```python
from build123d import *

# Parameters (mm, degrees)
ESBO_O2_R                = 1
RESSALTO_EXTRUS_O1_DEPTH = 1
RESSALTO_EXTRUS_O2_START = 1
ESBO_O4_R                = 1
RESSALTO_EXTRUS_O2_DEPTH = 1
CHANFRO1_SIZE            = 0.3
CHANFRO2_SIZE            = 0.3


with BuildPart() as part:
    # Esboço1 → Revolução2 (revolve)
    with BuildSketch(Plane.XY, mode=Mode.PRIVATE) as revolu_o2_sk:
        Polygon((-1, 5), (-1.5, 5), (-1.5, 0), (1.5, 0), (1.5, 5), (1, 5), (1, 4), (0, 4), (-1, 4), align=None)
    revolve(revolu_o2_sk.sketch.rotate(Axis((0, 0, 0), (1, 0, 0)), 90), axis=Axis((0, 0, 0), (1, 0, 0)))

    # Esboço2 → Ressalto-extrusão1 (add)
    with BuildSketch(Plane.ZY.offset(1.5)):
        Circle(ESBO_O2_R)
    extrude(amount=RESSALTO_EXTRUS_O1_DEPTH)

    # Esboço4 → Ressalto-extrusão2 (add)
    with BuildSketch(Plane(origin=(1.5, 0, 0), x_dir=(0, 0, -1), z_dir=(1, 0, 0)).offset(RESSALTO_EXTRUS_O2_START)):
        with Locations(Location((0, 0, 0), (0, 0, 180))):
            Circle(ESBO_O4_R)
    extrude(amount=-RESSALTO_EXTRUS_O2_DEPTH)

    # Chanfro1
    chanfro1_edges = [part.edges().sort_by_distance(p)[0] for p in [
        (-2.5, 0, -1),
    ]]
    chamfer(chanfro1_edges, length=CHANFRO1_SIZE)

    # Chanfro2
    chanfro2_edges = [part.edges().sort_by_distance(p)[0] for p in [
        (2.5, 0, -1),
    ]]
    chamfer(chanfro2_edges, length=CHANFRO2_SIZE)


solid = part.part
```
Verification items for the finished model (mm, model axes). A direction names the side the tool comes from. Round coordinates to 2 decimals unless told otherwise and drop trailing zeros. Write each loop counter-clockwise with the first axis right and the second up, starting at its lowest first coordinate (ties: lowest second). Pieces come first, ordered by that corner, then holes.
1. Draft check along X on faces 4 (the cylindrical face through (-0.014, 3.905, -0.867)), 5 (the flat face through (-1.5, -1.2, -0.1)), 6 (the flat face through (1.5, -1.2, 0.1)), 7 (the cylindrical face through (1.246, -0.22, -4.995)). Enter one of: +X half, -X half, draft (parallel to the pull), parting line (faces both ways), or undercut.
2. Section check C-C on x = 1.8. Enter the section's corners in (y, z).
3. Section check A-A on z = 0. Enter the section's corners in (x, y).
4. Section check D-D on z = 1.5. Enter the section's corners in (x, y).
5. Gauge pin test, flat ends, axial feed: P1, Ø1, axis at y = 2.5, z = 1, coming from the +X side; P2, Ø2, axis at x = 2, z = -3.5, coming from the -Y side; P3, Ø1, axis at x = -1.5, z = -3.5, coming from the -Y side. Record the tip position at first contact, or that the pin passes through.
6. Access from +Z, -Z, +X, -X, +Y, -Y to the whole of each face (thin tool, end or side, straight path). Record for faces 1 (the cylindrical face through (2, 1, 0)), 2 (the cylindrical face through (-1.254, -0.22, -4.995)), 3 (the cylindrical face through (-2, -1, 0)).
7. Scan lines: L1, parallel to X at y = -1.75, z = 4.25; L2, parallel to X at y = -1.75, z = -0.5; L3, parallel to Y at x = 1.3, z = 3. Record each from-to range of solid material in increasing order.
Answer:
1. face 4: undercut
1. face 5: -X half
1. face 6: +X half
1. face 7: draft
2. outline: circle Ø2 at (0, 0)
3. outline: (-2.5, -0.7) - (-2.2, -1) - (-1.5, -1) - (-1.5, -5) - (-1, -5) - (-1, -4) - (1, -4) - (1, -5) - (1.5, -5) - (1.5, -1) - (2.2, -1) - (2.5, -0.7) - (2.5, 0.7) - (2.2, 1) - (1.5, 1) - (1.5, 5) - (1, 5) - (1, 4) - (-1, 4) - (-1, 5) - (-1.5, 5) - (-1.5, 1) - (-2.2, 1) - (-2.5, 0.7) - close
4. outline: (-1.5, -4.77) - (-1, -4.77) - (-1, -3.71) - (1, -3.71) - (1, -4.77) - (1.5, -4.77) - (1.5, 4.77) - (1, 4.77) - (1, 3.71) - (-1, 3.71) - (-1, 4.77) - (-1.5, 4.77) - close
5. P1: stops at x = 1.5
5. P2: stops at y = -4.25
5. P3: stops at y = -4
6. face 1: +X
6. face 2: +X, -X
6. face 3: -X
7. L1: x = -1.5 to -1, 1 to 1.5
7. L2: x = -1.5 to 1.5
7. L3: y = -4 to 4
